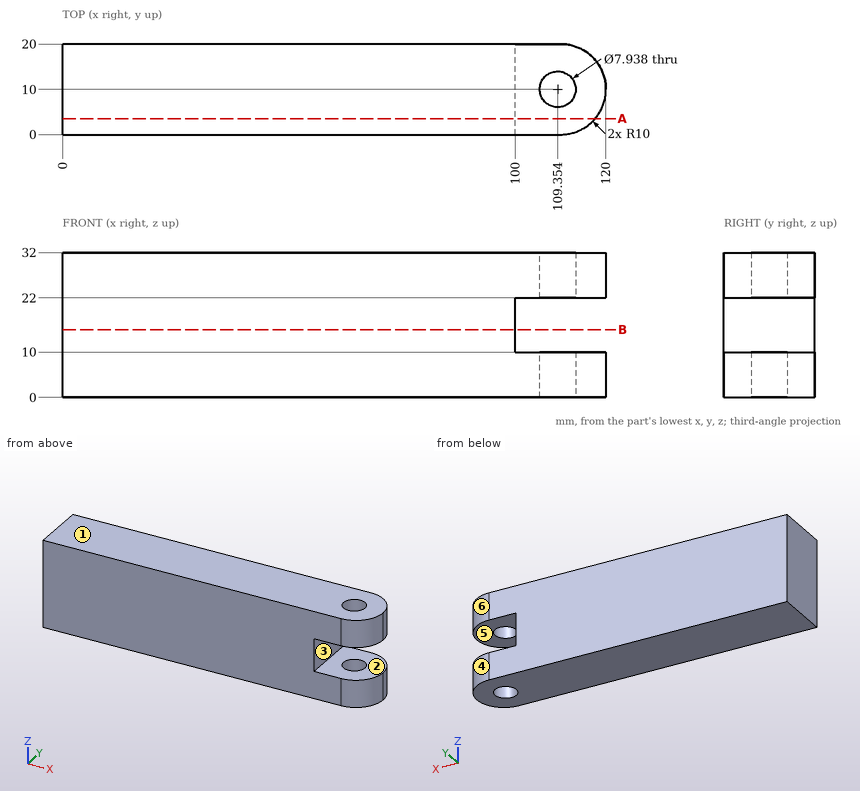
Part print with two shaded views. Sizes in mm from the minimum x, y, z corner. A direction names the side the tool comes from. Round coordinates to 2 decimals unless told otherwise and drop trailing zeros. Loops run counter-clockwise (first coordinate to the right, second up) from the corner with the lowest first, then second, coordinate; pieces in that order, holes last. Notation, with made-up numbers: (70.25, 87.25) - (124.25, 87.25) arc R19 cw to (124.25, 116.25) - close; hole circle Ø3 at (73.5, 52.5). An arc over 180 degrees is marked (long way). Answer as a JSON object with one key per item and string values.
Item 1: Band-saw the part on B-B on z = 15. List the corners of the cut face in (x, y).
Output:
{"outline": "(0, 0) - (100, 0) - (100, 20) - (0, 20) - close"}
Item 2: Tool access for the marked faces 5 and 6: list every direction of +Z, -Z, +X, -X, +Y, -Y with a clear straight run to the whole face (end or side of a thin tool).
Output:
{"face 5": "+X, +Y, -Y", "face 6": "+Z, -Z, +X, +Y"}
Item 3: Pin check, flat tips, straight feed: pin 1 (3.5 mm diameter, centred on y = 9, z = 15, fed in from +X); pin 2 (2 mm diameter, centred on y = 12, z = 10.5, fed in from +X) (1 decimal). Stop position of each tip, or through.
Output:
{"pin 1": "x = 100", "pin 2": "x = 119.9"}
Item 4: Wall check: L1, parallel to X at y = 9.75, z = 6.5 (1 decimal); L2, parallel to X at y = 2.5, z = 12.5; L3, parallel to X at y = 1.25, z = 27 (1 decimal). Give the ranges that are in metal, low to high.
Output:
{"L1": "0 to 105.4, 113.3 to 120", "L2": "0 to 100", "L3": "0 to 114.8"}
Item 5: Band-saw the part on A-A on y = 3.5. List the corners of the cut face in (x, z).
Output:
{"outline": "(0, 0) - (117.6, 0) - (117.6, 10) - (100, 10) - (100, 22) - (117.6, 22) - (117.6, 32) - (0, 32) - close"}
Item 6: Pull direction Z, two halves, no side cores. Call the marked faces 1, 2, 3 and 4: pulls with the +Z half, pulls with the -Z half, needs draft (parallel to the pull), parting line crosses it, or undercut.
Output:
{"face 1": "pulls with the +Z half", "face 2": "undercut", "face 3": "undercut", "face 4": "needs draft"}
